Here's how the part is built. I have some questions about the finished solid (model axes, mm). A direction names the side the tool comes from. Round coordinates to 2 decimals unless told otherwise and drop trailing zeros. Loops run counter-clockwise (first coordinate to the right, second up) from the corner with the lowest first, then second, coordinate; pieces in that order, holes last. Notation, with made-up numbers: M 34.25,56 L 39.25,56 A22 ccw 39.25,63 Z; hole C 19,59 d9. An arc over 180 degrees is marked long. Answer as a JSON object with one key per item and string values.
from build123d import *
from build123d.topology import SkipClean

# Parameters (mm, degrees)
CROQUIS1_W              = 8
CROQUIS1_H              = 30
SALIENTE_EXTRUIR1_DEPTH = 15
CORTAR_EXTRUIR1_DEPTH   = 34.778691508
SALIENTE_EXTRUIR2_DEPTH = 7.5
CROQUIS4_W              = 10
CROQUIS4_H              = 9
CORTAR_EXTRUIR2_DEPTH   = 10
CROQUIS5_R              = 1.6
CORTAR_EXTRUIR3_DEPTH   = 23.825424421
SALIENTE_EXTRUIR3_DEPTH = 3.5
REDONDEO1_R             = 1


with BuildPart() as part:
    # Croquis1 → Saliente-Extruir1 (new body)
    with BuildSketch(Plane(origin=(0, 0, 0), x_dir=(1, 0, 0), z_dir=(0, 1, 0))):
        Rectangle(CROQUIS1_W, CROQUIS1_H)
    extrude(amount=SALIENTE_EXTRUIR1_DEPTH)

    # Croquis2 → Cortar-Extruir1 (cut, through all)
    with BuildSketch(Plane.XY.offset(15)):
        Polygon((4, 15), (1, 0), (4, 0), align=None)
    extrude(amount=-CORTAR_EXTRUIR1_DEPTH, mode=Mode.SUBTRACT)

    # Croquis3 → Saliente-Extruir2 (add, symmetric)
    with BuildSketch(Plane.XY):
        Polygon((-14, 0), (-4, 0), (-4, 15), (-14, 5), align=None)
    extrude(amount=SALIENTE_EXTRUIR2_DEPTH, both=True)

    # Croquis4 → Cortar-Extruir2 (cut)
    with BuildSketch(Plane(origin=(0, 15, 0), x_dir=(1, 0, 0), z_dir=(0, 1, 0))):
        with Locations((-9, 0)):
            Rectangle(CROQUIS4_W, CROQUIS4_H)
    extrude(amount=-CORTAR_EXTRUIR2_DEPTH, mode=Mode.SUBTRACT)

    # Croquis5 → Cortar-Extruir3 (cut, through all)
    with BuildSketch(Plane(origin=(0, 5, 0), x_dir=(1, 0, 0), z_dir=(0, 1, 0))):
        with Locations(Location((-9, 0, 0), (0, 0, 270))):
            Circle(CROQUIS5_R)
    extrude(amount=-CORTAR_EXTRUIR3_DEPTH, mode=Mode.SUBTRACT)

    # Croquis6 → Saliente-Extruir3 (add)
    with SkipClean():  # the faces are left unmerged after this step: merging them gives an invalid solid
        with BuildSketch(Plane.XZ):
            with BuildLine():
                Line((-8.443223564, 1.5), (-4, 1.5))
                Line((-4, 1.5), (-4, -1.5))
                Line((-4, -1.5), (-8.443223564, -1.5))
                ThreePointArc((-8.443223564, -1.5), (-7.4, 0), (-8.443223564, 1.5))
            make_face()
            with BuildLine():
                Line((-14, -1.5), (-9.556776436, -1.5))
                ThreePointArc((-9.556776436, -1.5), (-10.6, 0), (-9.556776436, 1.5))
                Line((-9.556776436, 1.5), (-14, 1.5))
                Line((-14, 1.5), (-14, -1.5))
            make_face()
        extrude(amount=SALIENTE_EXTRUIR3_DEPTH)

    # Redondeo1
    # the kernel refuses this fillet: 1 mm, written as the material it takes off along each edge
    with BuildSketch(Plane(origin=(-8.443223564, 0, 1.5), x_dir=(1, 0, 0), z_dir=(0, -1, 0)), Plane(origin=(-9.556776436, 0, -1.5), x_dir=(-1, 0, 0), z_dir=(0, -1, 0))) as redondeo1_piece_1:
        with BuildLine():
            CenterArc((1.994693728, -1), REDONDEO1_R, 90, 101.087489211)
            ThreePointArc((1.01335905, -1.192307692), (0.662378184, -0.463823369), (0, 0))
            Line((0, 0), (1.994693728, 0))
        make_face()
    extrude(amount=8.48673432, mode=Mode.SUBTRACT)
    with BuildSketch(Plane(origin=(-8.443223564, 0, -1.5), x_dir=(1, 0, 0), z_dir=(0, -1, 0)), Plane(origin=(-9.556776436, 0, 1.5), x_dir=(-1, 0, 0), z_dir=(0, -1, 0))) as redondeo1_piece_2:
        with BuildLine():
            CenterArc((1.994693728, 1), REDONDEO1_R, 168.912510789, 101.087489211)
            ThreePointArc((1.01335905, 1.192307692), (0.662378184, 0.463823369), (0, 0))
            Line((0, 0), (1.994693728, 0))
        make_face()
    extrude(amount=8.48673432, mode=Mode.SUBTRACT)


solid = part.part
Item 1: For P1, Ø2.5, axis at x = -5.5, y = -1.5, coming from the -Z side; P2, Ø3, axis at x = -9, y = 8, coming from the +Z side; P3, Ø4.5, axis at x = -9, z = 1, coming from the +Y side; P4, Ø1.9, axis at x = -9, z = 0, coming from the +Y side, each with a flat end and sliding along its axis, tell me the tip position at first contact or that it passes through.
Solution:
{"P1": "stops at z = -1.5", "P2": "stops at z = 7.5", "P3": "stops at y = 5", "P4": "passes through"}
Item 2: If I drill on L1, parallel to Z at x = -9, y = 1.05; L2, parallel to Z at x = -4.5, y = 12.5; L3, parallel to Y at x = -1, z = 9.5, over which ranges is the centre line in solid material (lowest first)? Write a range as from..to.
Solution:
{"L1": "z = -7.5..-1.6, 1.6..7.5", "L2": "z = -7.5..-4.5, 4.5..7.5", "L3": "y = 0..15"}
Item 3: I want a section at D-D on y = 12.25. List the corners of the cut face in (x, z) for me, plus the area to 3 significant figures.
Solution:
{"outline": "M -6.75,-7.5 L -4,-7.5 L -4,-15 L 3.45,-15 L 3.45,15 L -4,15 L -4,7.5 L -6.75,7.5 L -6.75,4.5 L -4,4.5 L -4,-4.5 L -6.75,-4.5 Z", "area": "240 mm2"}
Item 4: I want a section at B-B on x = -6. List the corners of the cut face in (y, z) for me, plus the area to 4 significant figures.
Solution:
{"outline": "M -3.5,-1.5 L 0,-1.5 L 0,-7.5 L 13,-7.5 L 13,-4.5 L 5,-4.5 L 5,4.5 L 13,4.5 L 13,7.5 L 0,7.5 L 0,1.5 L -3.5,1.5 Z", "area": "133.5 mm2"}
Item 5: I want a section at A-A on x = -9. List the corners of the cut face in (y, z) for me, plus the area to 3 significant figures.
Solution:
{"outline": "M 0,-7.5 L 10,-7.5 L 10,-4.5 L 5,-4.5 L 5,-1.6 L 0,-1.6 Z; M 0,1.6 L 5,1.6 L 5,4.5 L 10,4.5 L 10,7.5 L 0,7.5 Z", "area": "89.0 mm2"}
Item 6: I want a section at C-C on z = 4. List the corners of the cut face in (x, y) for me, plus the area to 4 significant figures.
Solution:
{"outline": "M -14,0 L 1,0 L 4,15 L -4,15 L -4,5 L -14,5 Z", "area": "147.5 mm2"}
Item 7: We'd pull the mould along X, two halves only. Please class faces 1 (the face through (-12, -3.5, 0)), 2 (the face through (-7.228, -1.726, -1.126)), 3 (the face through (-4, 10, 0)): +X half, -X half, draft (parallel to the pull), parting line (faces both ways), or undercut.
Solution:
{"face 1": "draft", "face 2": "undercut", "face 3": "-X half"}
Item 8: For faces 4 (the face through (-4, 7, -11)), 5 (the face through (-8, 6, 7.5)), 6 (the face through (-7, 8, -4.5)), 7 (the face through (-13, -2, 1.5)), 8 (the face through (-4, -2, 0)), which set-ups out of +Z, -Z, +X, -X, +Y, -Y let a thin tool reach every point of the face, with its end or its side?
Solution:
{"face 4": "-Z, -X, +Y, -Y", "face 5": "+Z, -X, +Y, -Y", "face 6": "-X, +Y", "face 7": "+Z, +X, -X, -Y", "face 8": "+Z, -Z, +X, -Y"}
